Verification items for the finished model (mm, model axes). A direction names the side the tool comes from. Round coordinates to 2 decimals unless told otherwise and drop trailing zeros. Loops run counter-clockwise (first coordinate to the right, second up) from the corner with the lowest first, then second, coordinate; pieces in that order, holes last. Notation, with made-up numbers: M 10,-27.5 L 31,-27.5 A18 cw 31,7.5 Z; hole C 53.25,10.5 d7. An arc over 180 degrees is marked long. Answer as CSV lines item,"result".
```python
from build123d import *

# Parameters (mm, degrees)
SKETCH1_R           = 2.413
BOSS_EXTRUDE1_DEPTH = 22.225
SKETCH2_R           = 3.96875
BOSS_EXTRUDE2_DEPTH = 4.826
CUT_EXTRUDE1_DEPTH  = 3.81


with BuildPart() as part:
    # Sketch1 → Boss-Extrude1 (new body)
    with BuildSketch(Plane.XY):
        Circle(SKETCH1_R)
    extrude(amount=BOSS_EXTRUDE1_DEPTH)

    # Sketch2 → Boss-Extrude2 (add)
    with BuildSketch(Plane.XY.offset(22.225)):
        Circle(SKETCH2_R)
    extrude(amount=BOSS_EXTRUDE2_DEPTH)

    # Sketch3 → Cut-Extrude1 (cut)
    with BuildSketch(Plane.XY.offset(27.051)):
        Polygon((2.291358881, 0), (1.14567944, 1.984375), (-1.14567944, 1.984375), (-2.291358881, 0), (-1.14567944, -1.984375), (1.14567944, -1.984375), align=None)
    extrude(amount=-CUT_EXTRUDE1_DEPTH, mode=Mode.SUBTRACT)


solid = part.part
```
1) Section check B-B (x = 0). Record the cut outline in (y, z) (3 decimals).
Here are the results:
outline,"M -3.969,22.225 L -2.413,22.225 L -2.413,0 L 2.413,0 L 2.413,22.225 L 3.969,22.225 L 3.969,27.051 L 1.984,27.051 L 1.984,23.241 L -1.984,23.241 L -1.984,27.051 L -3.969,27.051 Z"
2) Material ranges on probe 1 along Z at (x, y) = (-0.5, -0.25); probe 2 along Z at (x, y) = (-3.5, 0.25) (3 decimals); probe 3 along Y at (x, z) = (0, 5.5), recorded low to high.
Here are the results:
probe 1,"z = 0 to 23.24"
probe 2,"z = 22.225 to 27.051"
probe 3,"y = -2.41 to 2.41"
3) Section check D-D (z = 16.5). Record the cut outline in (x, y).
Here are the results:
outline,"C 0,0 d4.83"
4) Go/stop test with a flat-tipped pin: pin 1 (1 mm diameter, centred on x = 1.5, z = 9.5, fed in from +Y). Record where the tip stops, or that it passes through.
Here are the results:
pin 1,"stops at y = 2.2"
5) Set-up check for faces 1 (the flat face through (-2, -1, 27.051)), 2 (the flat face through (-1.71, 1.01, 25.17)), 3 (the cylindrical face through (-1.915, -1.468, 10.957)): record each of +Z, -Z, +X, -X, +Y, -Y from which the full face is reachable in a straight line by a thin tool's end or side.
Here are the results:
face 1,"+Z, +X, -X, +Y, -Y"
face 2,"+Z"
face 3,"-Z"
6) Section check C-C (y = -1.5). Record the cut outline in (x, z) (3 decimals), plus the area to 3 significant figures.
Here are the results:
outline,"M -3.674,22.225 L -1.89,22.225 L -1.89,0 L 1.89,0 L 1.89,22.225 L 3.674,22.225 L 3.674,27.051 L 1.425,27.051 L 1.425,23.241 L -1.425,23.241 L -1.425,27.051 L -3.674,27.051 Z"
area,"109 mm^2"
7) Draft check along Y on faces 4 (the cylindrical face through (-0.86, -3.874, 24.604)), 5 (the flat face through (0, 0, 0)), 6 (the flat face through (0, 1.984, 25)). Enter one of: +Y half, -Y half, draft (parallel to the pull), parting line (faces both ways), or undercut.
Here are the results:
face 4,"parting line"
face 5,"draft"
face 6,"undercut"
8) Section check A-A (z = 24). Record the cut outline in (x, y).
Here are the results:
outline,"C 0,0 d7.94; hole M -2.29,0 L -1.15,-1.98 L 1.15,-1.98 L 2.29,0 L 1.15,1.98 L -1.15,1.98 Z"
